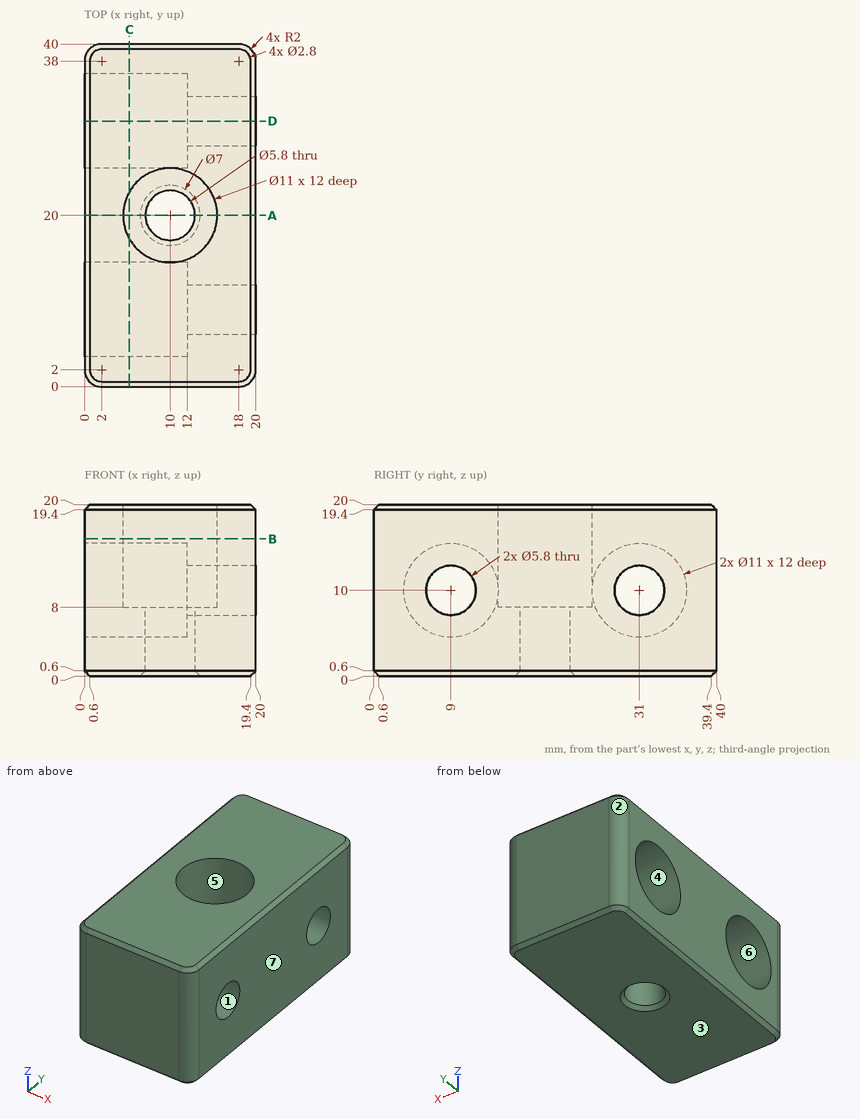
Input: dimensioned drawing with shaded views. Units: mm. Origin: part minimum x, y, z. A direction names the side the tool comes from. Coordinates: 2 decimals unless noted, no trailing zeros. Loops run counter-clockwise (first coordinate to the right, second up) from the corner with the lowest first, then second, coordinate; pieces in that order, holes last. Notation, with made-up numbers: M 3.25,57 L 55.25,57 A23 ccw 55.25,92 Z; hole C 88.25,-36 d11. An arc over 180 degrees is marked long. One line per item, written item: value.
(1) Section C-C (x = 5.25). Output: boundary loops of the cut face in (y, z).
Filled in:
outline: M 0,0.6 L 0.6,0 L 39.4,0 L 40,0.6 L 40,19.4 L 39.4,20 L 22.77,20 L 22.77,8 L 17.23,8 L 17.23,20 L 0.6,20 L 0,19.4 Z; hole C 9,10 d11; hole C 31,10 d11
(2) Pin query (flat end, axial travel): pin 1 (12 mm diameter, centred on y = 24.5, z = 9.5, fed in from -X); pin 2 (9 mm diameter, centred on y = 9, z = 10, fed in from -X). Return the tip coordinate at first contact, or that it passes through.
Filled in:
pin 1: x = 0
pin 2: x = 12
(3) Line query: line 1 along Y through (x, z) = (4.25, 10); line 2 along Y through (x, z) = (16.75, 10); line 3 along Z through (x, y) = (15.5, 9). Output: solid intervals per line, ascending. Write a range as from..to.
Filled in:
line 1: 0..3.5, 14.5..25.5, 36.5..40
line 2: 0..6.1, 11.9..28.1, 33.9..40
line 3: 0..7.1, 12.9..20
(4) Section A-A (y = 20). Output: boundary loops of the cut face in (x, z).
Filled in:
outline: M 0,0.6 L 0.6,0 L 6.5,0 L 7.1,0.6 L 7.1,8 L 4.5,8 L 4.5,20 L 0.6,20 L 0,19.4 Z; M 12.9,0.6 L 13.5,0 L 19.4,0 L 20,0.6 L 20,19.4 L 19.4,20 L 15.5,20 L 15.5,8 L 12.9,8 Z
(5) Section B-B (z = 16). Output: boundary loops of the cut face in (x, y).
Filled in:
outline: M 0,2 A2 ccw 2,0 L 18,0 A2 ccw 20,2 L 20,38 A2 ccw 18,40 L 2,40 A2 ccw 0,38 Z; hole C 10,20 d11
(6) Reachability of the marked faces 5, 6 and 7 from +Z, -Z, +X, -X, +Y, -Y: full face, straight path, thin tool, end or side. Return the list, or none.
Filled in:
face 5: +Z
face 6: -X
face 7: +Z, -Z, +X, +Y, -Y
(7) Section D-D (y = 31). Output: boundary loops of the cut face in (x, z).
Filled in:
outline: M 0,0.6 L 0.6,0 L 19.4,0 L 20,0.6 L 20,7.1 L 12,7.1 L 12,4.5 L 0,4.5 Z; M 0,15.5 L 12,15.5 L 12,12.9 L 20,12.9 L 20,19.4 L 19.4,20 L 0.6,20 L 0,19.4 Z
(8) Pull-direction query (Y, two-part tool) for the marked faces 1, 2, 3 and 4; classes: +Y half, -Y half, draft (parallel to the pull), parting line (faces both ways), or undercut.
Filled in:
face 1: undercut
face 2: +Y half
face 3: draft
face 4: undercut
